For this review, take the finished solid that the model builds, in its own axes (mm). Round coordinates to 2 decimals unless told otherwise and drop trailing zeros. Order: outer loops, then holes, each group sorted by start corner. A loop starts at its lowest first (then second) coordinate and runs counter-clockwise, first axis right, second up. Notation, with made-up numbers: (20.5, 34.5) - (40.5, 34.5) arc R20 cw to (40.5, 62.5) - close; hole circle Ø2 at (-5, 75). An arc over 180 degrees is marked (long way). One line per question, with ' | ' between items.
```python
from build123d import *

# Parameters (mm, degrees)
SKETCH1_R           = 1.5
SKETCH1_R_2         = 8
BOSS_EXTRUDE6_DEPTH = 2


with BuildPart() as part:
    # Sketch1 → Boss-Extrude6 (new body)
    with BuildSketch(Plane(origin=(0, 0, 0), x_dir=(1, 0, 0), z_dir=(0, 1, 0))):
        with BuildLine():
            ThreePointArc((-42.892787305, 62.910010988), (-49.963855117, 59.981078799), (-52.892787305, 52.910010988))
            Line((-52.892787305, 52.910010988), (-52.892787305, 24.160010988))
            Line((-52.892787305, 24.160010988), (-52.892787305, 1.660010988))
            Line((-52.892787305, 1.660010988), (-52.892787305, -27.089989012))
            ThreePointArc((-52.892787305, -27.089989012), (-49.963855117, -34.161056824), (-42.892787305, -37.089989012))
            Line((-42.892787305, -37.089989012), (137.102440603, -37.089989012))
            ThreePointArc((137.102440603, -37.089989012), (144.173508414, -34.161056824), (147.102440603, -27.089989012))
            Line((147.102440603, -27.089989012), (147.102440603, 1.660010988))
            Line((147.102440603, 1.660010988), (147.102440603, 24.160010988))
            Line((147.102440603, 24.160010988), (147.102440603, 52.910010988))
            ThreePointArc((147.102440603, 52.910010988), (144.173508414, 59.981078799), (137.102440603, 62.910010988))
            Line((137.102440603, 62.910010988), (61.731596977, 62.910010988))
            ThreePointArc((61.731596977, 62.910010988), (60.27668109, 63.779465055), (59.705316327, 65.375169578))
            Line((59.705316327, 65.375169578), (59.705316327, 69.910696544))
            ThreePointArc((59.705316327, 69.910696544), (77.704972023, 87.799364481), (59.927976193, 105.909319341))
            Line((59.927976193, 105.909319341), (59.483635762, 105.909331429))
            Line((59.483635762, 105.909331429), (34.505806024, 105.910010948))
            Line((34.505806024, 105.910010948), (34.504826649, 105.910010974))
            ThreePointArc((34.504826649, 105.910010974), (16.504826662, 87.910010988), (34.504826649, 69.910011001))
            Line((34.504826649, 69.910011001), (34.504826649, 65.374484021))
            ThreePointArc((34.504826649, 65.374484021), (33.890722022, 63.738204886), (32.35168701, 62.910010988))
            Line((32.35168701, 62.910010988), (-42.892787305, 62.910010988))
        make_face()
        with Locations(Location((-42.892787305, -27.089989012, 0), (0, 0, 270))):
            Circle(SKETCH1_R, mode=Mode.SUBTRACT)
        with Locations(Location((137.102440603, -27.089989012, 0), (0, 0, 270))):
            Circle(SKETCH1_R, mode=Mode.SUBTRACT)
        with Locations(Location((-42.892787305, 52.910010988, 0), (0, 0, 270))):
            Circle(SKETCH1_R, mode=Mode.SUBTRACT)
        with Locations(Location((34.504826649, 87.910010988, 0), (0, 0, 270))):
            Circle(SKETCH1_R_2, mode=Mode.SUBTRACT)
        with Locations(Location((137.102440603, 52.612926661, 0), (0, 0, 270))):
            Circle(SKETCH1_R, mode=Mode.SUBTRACT)
        with Locations(Location((59.705316327, 87.910696544, 0), (0, 0, 270))):
            Circle(SKETCH1_R_2, mode=Mode.SUBTRACT)
    extrude(amount=BOSS_EXTRUDE6_DEPTH)


solid = part.part
```
(1) We need section C-C on z = -83.5. State the section outline as (x, y) points, plus the area to 3 significant figures.
Output values:
outline: (17.05, 0) - (27.83, 0) - (27.83, 2) - (17.05, 2) - close; (41.18, 0) - (53.03, 0) - (53.03, 2) - (41.18, 2) - close; (66.38, 0) - (77.16, 0) - (77.16, 2) - (66.38, 2) - close | area: 66.8 mm^2
(2) Insertion check: pin 1 (3.5 mm diameter, centred on x = -42.89, z = 27.09, fed in from -Y). The pin has a flat end and moves straight along its axis. Give the tip position at first contact, or say it passes through.
Output values:
pin 1: y = 0
(3) We need section B-B on x = 57. State the section outline as (y, z) points, plus the area to 3 significant figures.
Output values:
outline: (0, -105.91) - (2, -105.91) - (2, -95.44) - (0, -95.44) - close; (0, -80.38) - (2, -80.38) - (2, 37.09) - (0, 37.09) - close | area: 256 mm^2
(4) We need section A-A on y = 1.05. Give the number of separate pieces and of enclosed holes in the cut face, plus the area to 3 significant figures.
Output values:
separate pieces: 1 | enclosed holes: 6 | area: 21,600 mm^2
(5) We need section D-D on x = 90.5. State the section outline as (y, z) points.
Output values:
outline: (0, -62.91) - (2, -62.91) - (2, 37.09) - (0, 37.09) - close
(6) Mouldability with a two-part tool opening along Z and no side actions: class faces 1 (the cylindrical face through (29.64, 0.99, -94.26)), 2 (the flat face through (46, 2, -20)), 3 (the cylindrical face through (144.251, 0.986, -59.903)) as released by +Z, released by -Z, zero draft, split by the parting line, or undercut.
Output values:
face 1: undercut | face 2: zero draft | face 3: released by -Z
(7) For probe 1 along X at (y, z) = (1.95, -87.5); probe 2 along X at (y, z) = (1.1, -91.5); probe 3 along Z at (x, y) = (-7, 0.4), list the stretches that pass through material, from the lowest coordinate up. Write a range as [from, to].
Output values:
probe 1: [16.51, 26.52], [42.49, 51.72], [67.69, 77.7] | probe 2: [16.87, 27.36], [41.65, 52.56], [66.85, 77.34] | probe 3: [-62.91, 37.09]
